Model file for the job. Use its own axes, mm. A direction names the side the tool comes from. Round coordinates to 2 decimals unless told otherwise and drop trailing zeros. Order: outer loops, then holes, each group sorted by start corner. A loop starts at its lowest first (then second) coordinate and runs counter-clockwise, first axis right, second up. Notation, with made-up numbers: (48, 78) -> (101, 78) arc R25 cw to (101, 94) -> close; hole circle Ø5 at (14.5, 78). An arc over 180 degrees is marked (long way). Put each result on its own line as item: value. Start each with the question number.
Q1. Cut at C-C, the plane x = 19. List the corners of the cut face in (y, z).
Q2. Pull direction Y, two halves, no side cores. Call faces 1 (the face through (18, 6.952, 12)), 2 (the face through (-1, 20, 4)), 3 (the face through (-3, -6.272, 12)), 4 (the face through (-26, 1, 10)): released by +Y, released by -Y, zero draft, split by the parting line, or undercut.
Q3. Probe L1, parallel to Z at x = 30.5, y = 13.5; L2, parallel to Y at x = 40, z = 11.5; L3, parallel to X at y = 10, z = 8.75. List the from-to ranges inside material, lowest first.
Q4. Flat gauge pins, fed straight in: P1, Ø1.2, axis at y = -4, z = 12.5, coming from the -X side; P2, Ø1, axis at x = -43, z = 11.5, coming from the -Y side; P3, Ø1.1, axis at x = -46, z = 13, coming from the +Y side. Where does each tip first touch, or does it go through?
Q5. Cut at B-B, the plane y = -9.5. List the corners of the cut face in (x, z), and give its area (3 significant figures).
Q6. 3-axis set-ups, long thin cutter, end or side, ignore diameter. For faces 5 (the face through (12.028, 1, 12)), 6 (the face through (29, -2.109, 12)), 7 (the face through (42, -6.272, 12)), 8 (the face through (-38.726, 5.326, 12.465)): which of +Z, -Z, +X, -X, +Y, -Y reach the whole face in a straight line?
Q7. Cut at A-A, the plane x = 39.5. List the corners of the cut face in (y, z).
Autodesk Inventor part; units mm, degrees
ref_plane "Plano de trabajo1" through (0, 0, 10) normal (0, 0, 1) x (1, 0, 0)
ref_plane "YZ Plane" through (0, 0, 0) normal (1, 0, 0) x (0, 1, 0)
ref_plane "XZ Plane" through (0, 0, 0) normal (0, 1, 0) x (-1, 0, 0)
sketch "Boceto1" plane through (0, 0, 0) normal (0, 0, 1) x (1, 0, 0)
  line L0 (0, 0) -> (-60, 0) construction
  line L1 (-60, 0) -> (-60, 20) construction
  line L2 (-60, 20) -> (60, 20)
  line L3 (60, 20) -> (60, -20)
  line L4 (60, -20) -> (-60, -20)
  line L5 (-60, -20) -> (-60, 20)
  dimension "d0" = 60
  dimension "d1" = 20
  dimension "d2" = 120
  dimension "d3" = 40
extrude "Extrusión1" add sketch "Boceto1" along normal blind 10
fillet "Empalme1" radius 2 4 edges at (0, 20, 10) (60, 0, 10) (0, -20, 10) (-60, 0, 10)
ref_plane "Plano de trabajo1" through (0, 0, 10) normal (0, 0, 1) x (1, 0, 0)
sketch "Boceto2" plane through (0, 0, 10) normal (0, 0, 1) x (1, 0, 0)
  line L0 (-47.1397, 9.0462) -> (47.4717, 9.0462) construction
  line L1 (47.4717, 9.0462) -> (47.4717, -9.0462) construction
  line L2 (47.4717, -9.0462) -> (-47.1397, -9.0462) construction
  line L3 (-47.1397, -9.0462) -> (-47.1397, 9.0462) construction
  line L4 (-60, 20) -> (-60, -20) construction
  line L5 (-60, 0) -> (-47.3055, 0) construction
  line L6 (60, -20) -> (60, 20) construction
  line L7 (-34.503, 8.7278) -> (-39.7806, 0.3033)
  line L8 (-39.7806, 0.3033) -> (-39.7806, -6.2722)
  line L9 (-39.7806, -6.2722) -> (-41.7765, -6.2722)
  line L10 (-41.7765, -6.2722) -> (-41.7765, 0.0952)
  line L11 (-41.7765, 0.0952) -> (-47.0785, 8.7278)
  line L12 (-47.0785, 8.7278) -> (-44.8622, 8.7278)
  line L13 (-44.8622, 8.7278) -> (-40.7724, 2.0176)
  line L14 (-40.7724, 2.0176) -> (-36.6214, 8.7278)
  line L15 (-36.6214, 8.7278) -> (-34.503, 8.7278)
  spline S0 degree 2 poles (-21.254, 7.0135) (-20.3357, 5.9972) (-19.3561, 3.0829) (-19.3561, 1.2217) knots 0 0 0 1 2 2 2
  spline S1 degree 2 poles (-19.3561, 1.2217) (-19.3561, -0.6273) (-20.3479, -3.5661) (-21.254, -4.5457) knots 0 0 0 1 2 2 2
  spline S2 degree 2 poles (-21.254, -4.5457) (-22.1724, -5.562) (-24.7071, -6.5906) (-26.3234, -6.5906) knots 0 0 0 1 2 2 2
  spline S3 degree 2 poles (-26.3234, -6.5906) (-27.903, -6.5906) (-30.4867, -5.5375) (-31.3928, -4.5457) knots 0 0 0 1 2 2 2
  spline S4 degree 2 poles (-31.3928, -4.5457) (-32.2989, -3.5416) (-33.2785, -0.6395) (-33.2785, 1.2217) knots 0 0 0 1 2 2 2
  spline S5 degree 2 poles (-33.2785, 1.2217) (-33.2785, 3.0584) (-32.3112, 5.9727) (-31.3806, 7.0135) knots 0 0 0 1 2 2 2
  spline S6 degree 2 poles (-31.3806, 7.0135) (-30.4989, 7.9931) (-27.8785, 9.0462) (-26.3234, 9.0462) knots 0 0 0 1 2 2 2
  spline S7 degree 2 poles (-26.3234, 9.0462) (-24.7071, 9.0462) (-22.1479, 7.9931) (-21.254, 7.0135) knots 0 0 0 1 2 2 2
  spline S8 degree 2 poles (-21.4254, 1.2217) (-21.4254, 4.1482) (-24.0459, 7.3197) (-26.3112, 7.3197) knots 0 0 0 1 2 2 2
  spline S9 degree 2 poles (-26.3112, 7.3197) (-28.601, 7.3197) (-31.2091, 4.1482) (-31.2091, 1.2217) knots 0 0 0 1 2 2 2
  spline S10 degree 2 poles (-31.2091, 1.2217) (-31.2091, -1.7293) (-28.552, -4.864) (-26.3112, -4.864) knots 0 0 0 1 2 2 2
  spline S11 degree 2 poles (-26.3112, -4.864) (-24.0703, -4.864) (-21.4254, -1.7293) (-21.4254, 1.2217) knots 0 0 0 1 2 2 2
  spline S12 degree 2 poles (-5.2867, -1.9865) (-5.2867, -2.8681) (-6.1071, -4.5824) (-6.8418, -5.1701) knots 0 0 0 1 2 2 2
  spline S13 degree 2 poles (-6.8418, -5.1701) (-7.6499, -5.8191) (-9.7928, -6.5416) (-11.2989, -6.5416) knots 0 0 0 1 2 2 2
  spline S14 degree 2 poles (-11.2989, -6.5416) (-12.9275, -6.5416) (-15.5234, -5.9416) (-16.8581, -5.3416) knots 0 0 0 1 2 2 2
  line L16 (-16.8581, -5.3416) -> (-16.8581, -2.8436)
  line L17 (-16.8581, -2.8436) -> (-16.7112, -2.8436)
  spline S15 degree 2 poles (-16.7112, -2.8436) (-15.5724, -3.7865) (-12.5969, -4.815) (-11.2744, -4.815) knots 0 0 0 1 2 2 2
  spline S16 degree 2 poles (-11.2744, -4.815) (-9.4254, -4.815) (-7.3561, -3.4314) (-7.3561, -2.2681) knots 0 0 0 1 2 2 2
  spline S17 degree 2 poles (-7.3561, -2.2681) (-7.3561, -1.2763) (-8.3357, -0.3334) (-9.3397, -0.064) knots 0 0 0 1 2 2 2
  spline S18 degree 2 poles (-9.3397, -0.064) (-10.0867, 0.1319) (-11.8622, 0.4013) (-12.8418, 0.5972) knots 0 0 0 1 2 2 2
  spline S19 degree 2 poles (-12.8418, 0.5972) (-14.8499, 1.0258) (-16.7724, 3.0707) (-16.7724, 4.7115) knots 0 0 0 1 2 2 2
  spline S20 degree 2 poles (-16.7724, 4.7115) (-16.7724, 6.585) (-13.5887, 8.9972) (-11.1275, 8.9972) knots 0 0 0 1 2 2 2
  spline S21 degree 2 poles (-11.1275, 8.9972) (-9.5479, 8.9972) (-6.903, 8.3972) (-5.8867, 7.9441) knots 0 0 0 1 2 2 2
  line L18 (-5.8867, 7.9441) -> (-5.8867, 5.5931)
  line L19 (-5.8867, 5.5931) -> (-6.0336, 5.5931)
  spline S22 degree 2 poles (-6.0336, 5.5931) (-6.8908, 6.3156) (-9.6826, 7.2707) (-11.152, 7.2707) knots 0 0 0 1 2 2 2
  spline S23 degree 2 poles (-11.152, 7.2707) (-12.7561, 7.2707) (-14.703, 5.9482) (-14.703, 4.8952) knots 0 0 0 1 2 2 2
  spline S24 degree 2 poles (-14.703, 4.8952) (-14.703, 3.9645) (-13.7357, 2.8992) (-12.5112, 2.6176) knots 0 0 0 1 2 2 2
  spline S25 degree 2 poles (-12.5112, 2.6176) (-11.8622, 2.4707) (-9.4867, 2.0666) (-8.654, 1.8584) knots 0 0 0 1 2 2 2
  spline S26 degree 2 poles (-8.654, 1.8584) (-6.9765, 1.4176) (-5.2867, -0.3824) (-5.2867, -1.9865) knots 0 0 0 1 2 2 2
  line L20 (9.7501, -6.2722) -> (7.6317, -6.2722)
  line L21 (7.6317, -6.2722) -> (6.1623, -2.1089)
  line L22 (6.1623, -2.1089) -> (-0.3642, -2.1089)
  line L23 (-0.3642, -2.1089) -> (-1.8214, -6.2722)
  line L24 (-1.8214, -6.2722) -> (-3.8418, -6.2722)
  line L25 (-3.8418, -6.2722) -> (1.6194, 8.7278)
  line L26 (1.6194, 8.7278) -> (4.2888, 8.7278)
  line L27 (4.2888, 8.7278) -> (9.7501, -6.2722)
  line L28 (5.5378, -0.3824) -> (2.9052, 6.989)
  line L29 (2.9052, 6.989) -> (0.2603, -0.3824)
  line L30 (0.2603, -0.3824) -> (5.5378, -0.3824)
  line L31 (21.6031, 6.9523) -> (14.0235, 6.9523)
  line L32 (14.0235, 6.9523) -> (14.0235, 2.7278)
  line L33 (14.0235, 2.7278) -> (20.5378, 2.7278)
  line L34 (20.5378, 2.7278) -> (20.5378, 0.9523)
  line L35 (20.5378, 0.9523) -> (14.0235, 0.9523)
  line L36 (14.0235, 0.9523) -> (14.0235, -6.2722)
  line L37 (14.0235, -6.2722) -> (12.0276, -6.2722)
  line L38 (12.0276, -6.2722) -> (12.0276, 8.7278)
  line L39 (12.0276, 8.7278) -> (21.6031, 8.7278)
  line L40 (21.6031, 8.7278) -> (21.6031, 6.9523)
  line L41 (35.7092, -6.2722) -> (33.5909, -6.2722)
  line L42 (33.5909, -6.2722) -> (32.1215, -2.1089)
  line L43 (32.1215, -2.1089) -> (25.595, -2.1089)
  line L44 (25.595, -2.1089) -> (24.1378, -6.2722)
  line L45 (24.1378, -6.2722) -> (22.1174, -6.2722)
  line L46 (22.1174, -6.2722) -> (27.5786, 8.7278)
  line L47 (27.5786, 8.7278) -> (30.248, 8.7278)
  line L48 (30.248, 8.7278) -> (35.7092, -6.2722)
  line L49 (31.497, -0.3824) -> (28.8643, 6.989)
  line L50 (28.8643, 6.989) -> (26.2194, -0.3824)
  line L51 (26.2194, -0.3824) -> (31.497, -0.3824)
  line L52 (48.6888, 6.9523) -> (43.3256, 6.9523)
  line L53 (43.3256, 6.9523) -> (43.3256, -6.2722)
  line L54 (43.3256, -6.2722) -> (41.3297, -6.2722)
  line L55 (41.3297, -6.2722) -> (41.3297, 6.9523)
  line L56 (41.3297, 6.9523) -> (35.9664, 6.9523)
  line L57 (35.9664, 6.9523) -> (35.9664, 8.7278)
  line L58 (35.9664, 8.7278) -> (48.6888, 8.7278)
  line L59 (48.6888, 8.7278) -> (48.6888, 6.9523)
  point P0 (0, 0)
  dimension "d8" = 94.6114
  dimension "d9" = 12.6945
  dimension "d10" = 12.5283
extrude "Extrusión2" add sketch "Boceto2" along normal blind 5
properties part number "Repujado 1"
Ans:
1. outline: (-20, 0) -> (20, 0) -> (20, 8) arc R2 ccw to (18, 10) -> (8.73, 10) -> (8.73, 15) -> (6.95, 15) -> (6.95, 10) -> (2.73, 10) -> (2.73, 15) -> (0.95, 15) -> (0.95, 10) -> (-18, 10) arc R2 ccw to (-20, 8) -> close
2. face 1: undercut
2. face 2: released by +Y
2. face 3: released by -Y
2. face 4: undercut
3. L1: z = 0 to 10
3. L2: y = 6.95 to 8.73
3. L3: x = -59.85 to 59.85
4. P1: stops at x = -41.78
4. P2: stops at y = 1.27
4. P3: stops at y = 8.73
5. outline: (-60, 0) -> (60, 0) -> (60, 8) arc R2 ccw to (58, 10) -> (-58, 10) arc R2 ccw to (-60, 8) -> close
5. area: 1,200 mm^2
6. face 5: +Z, +Y, -Y
6. face 6: +Z, -Y
6. face 7: +Z, +X, -Y
6. face 8: +Z, +Y
7. outline: (-20, 0) -> (20, 0) -> (20, 8) arc R2 ccw to (18, 10) -> (8.73, 10) -> (8.73, 15) -> (6.95, 15) -> (6.95, 10) -> (-18, 10) arc R2 ccw to (-20, 8) -> close
